```python
from build123d import *

# Parameters (mm, degrees)
F1_R      = 7.62
F2_DEPTH  = 8.9916
F3_R      = 3.175
F4_DEPTH  = 18.5
F7_DEPTH  = 21.5
F5_R      = 1.4351
F8_DEPTH  = 25.4
F11_DEPTH = 20
F12_R     = 2.54
F13_SIZE  = 2.54
F6_R      = 30.2514
F14_DEPTH = 2.032
F16_R     = 30.2514
F17_DEPTH = 2.032
F18_R     = 5.9079449729
F19_DEPTH = 3.81
F20_R     = 3.175
F20_R_2   = 1.016
F21_DEPTH = 20


# Not quite as in the source:
# - a feature of the source that left no trace in its solid (it failed there, or was rolled back) is left out
# - a feature names something its author has since deleted; it is built from what else it names


with BuildPart() as f2:
    # F1 (on Top) → F2 (new body)
    with BuildSketch(Plane.XY):
        with BuildLine():
            Line((14.3891, -27.8892), (14.3891, 5.7461149649))
            ThreePointArc((14.3891, 5.7461149649), (0, 15.494), (-14.3891, 5.7461149649))
            Line((-14.3891, 5.7461149649), (-14.3891, -27.8892))
            Line((-14.3891, -27.8892), (14.3891, -27.8892))
        make_face()
        Circle(F1_R, mode=Mode.SUBTRACT)
    extrude(amount=F2_DEPTH)


with BuildPart() as f4:
    # F3 (on Top) → F4 (new body)
    with BuildSketch(Plane.XY):
        Circle(F3_R)
    extrude(amount=F4_DEPTH)


with BuildPart() as f7:
    # F0 (on Top) → F7 (new body)
    with BuildSketch(Plane.XY):
        with BuildLine():
            Line((32.2834, -36.9807843447), (32.2834, 0))
            ThreePointArc((32.2834, 0), (0, 32.2834), (-32.2834, 0))
            Line((-32.2834, 0), (-32.2834, -36.9807843447))
            ThreePointArc((-32.2834, -36.9807843447), (-28.5636561211, -45.9610404657), (-19.5834, -49.6807843447))
            Line((-19.5834, -49.6807843447), (19.5834, -49.6807843447))
            ThreePointArc((19.5834, -49.6807843447), (28.5636561211, -45.9610404657), (32.2834, -36.9807843447))
        make_face()
    extrude(amount=F7_DEPTH)

    # F5 (on Top) → F8 (cut)
    with BuildSketch(Plane.XY):
        with Locations((-23.0124, 0)):
            Circle(F5_R)
        with Locations((23.0124, 0)):
            Circle(F5_R)
    extrude(amount=F8_DEPTH, mode=Mode.SUBTRACT)


with BuildPart() as f11_tool:
    # F10 (on Top) → F11 (new body)
    with BuildSketch(Plane.XY):
        with BuildLine():
            Line((-23.5020610966, -3.7882152164), (-27.6819982204, -3.7882152164))
            ThreePointArc((-27.6819982204, -3.7882152164), (-0.010778614, -27.9399979209), (27.6790671673, -3.8095722529))
            Line((27.6790671673, -3.8095722529), (23.0213215121, -3.8095722529))
            ThreePointArc((23.0213215121, -3.8095722529), (19.1556447136, -0.1037564295), (22.8138242261, 3.8070300236))
            ThreePointArc((22.8138242261, 3.8070300236), (22.9642316699, 3.81), (23.1146391137, 3.8070300236))
            Line((23.1146391137, 3.8070300236), (27.6794169447, 3.8070300236))
            ThreePointArc((27.6794169447, 3.8070300236), (-0.0092095477, 27.9399984822), (-27.6819206668, 3.7887818881))
            Line((-27.6819206668, 3.7887818881), (-23.4967496803, 3.7887818881))
            ThreePointArc((-23.4967496803, 3.7887818881), (-19.3067133937, 0.4041926109), (-22.688364657, -3.7882152164))
            ThreePointArc((-22.688364657, -3.7882152164), (-23.0952128768, -3.81), (-23.5020610966, -3.7882152164))
        make_face()
        with BuildLine():
            ThreePointArc((27.6790671673, -3.8095722529), (-0.010778614, -27.9399979209), (-27.6819982204, -3.7882152164))
            Line((-27.6819982204, -3.7882152164), (-27.6819982204, -34.7421456456))
            ThreePointArc((-27.6819982204, -34.7421456456), (-24.7062031172, -41.9263505425), (-17.5219982204, -44.9021456456))
            Line((-17.5219982204, -44.9021456456), (17.5190671673, -44.9021456456))
            ThreePointArc((17.5190671673, -44.9021456456), (24.7032720641, -41.9263505425), (27.6790671673, -34.7421456456))
            Line((27.6790671673, -34.7421456456), (27.6790671673, -3.8095722529))
        make_face()
        with BuildLine():
            Line((-22.688364657, -3.7882152164), (-23.5020610966, -3.7882152164))
            ThreePointArc((-23.5020610966, -3.7882152164), (-23.0952128768, -3.81), (-22.688364657, -3.7882152164))
        make_face()
        with BuildLine():
            ThreePointArc((23.1146391137, 3.8070300236), (22.9642316699, 3.81), (22.8138242261, 3.8070300236))
            Line((22.8138242261, 3.8070300236), (23.1146391137, 3.8070300236))
        make_face()
    extrude(amount=F11_DEPTH)


with BuildPart() as f2_1:
    add(f2.part)

    # F11: cut by f11_tool
    add(f11_tool.part, mode=Mode.SUBTRACT)


with BuildPart() as f4_1:
    add(f4.part)

    # F11: cut by f11_tool
    add(f11_tool.part, mode=Mode.SUBTRACT)


with BuildPart() as f7_1:
    add(f7.part)

    # F11: cut by f11_tool
    add(f11_tool.part, mode=Mode.SUBTRACT)

    # F12
    f12_edges = [f7_1.edges().sort_by_distance(p)[0] for p in [
        (0, 32.2834, 21.5),
        (32.2834, -18.490392, 21.5),
        (28.563656, -45.96104, 21.5),
        (0, -49.680784, 21.5),
        (-32.2834, -18.490392, 21.5),
        (-28.563656, -45.96104, 21.5),
    ]]
    fillet(f12_edges, radius=F12_R)

    # F13
    f13_edges = [f7_1.edges().sort_by_distance(p)[0] for p in [
        (-24.4475, 0, 21.5),
        (21.5773, 0, 21.5),
    ]]
    chamfer(f13_edges, length=F13_SIZE)

    # F6 (on Top) → F14 (cut)
    with BuildSketch(Plane.XY):
        Circle(F6_R)
    extrude(amount=F14_DEPTH, mode=Mode.SUBTRACT)

    # F16 (on Top) + F6 (on Top) → F17 (cut)
    with BuildSketch(Plane.XY):
        Circle(F16_R)
    with BuildSketch(Plane.XY):
        Circle(F6_R)
    extrude(amount=F17_DEPTH, mode=Mode.SUBTRACT)

    # F18 (on face) → F19 (cut)
    with BuildSketch(Plane.XZ.offset(49.6807843447)):
        with Locations((0, 9.48)):
            Circle(F18_R)
    extrude(amount=-F19_DEPTH, mode=Mode.SUBTRACT)

    # F20 (on face) → F21 (join, through all)
    with BuildSketch(Plane(origin=(0, 0, 20), x_dir=(1, 0, 0), z_dir=(0, 0, -1))):
        with Locations((17.5190671673, 34.7421456456)):
            Circle(F20_R)
        with Locations((17.5190671673, 34.7421456456)):
            Circle(F20_R_2, mode=Mode.SUBTRACT)
        with Locations((-17.5219982204, 34.7421456456)):
            Circle(F20_R)
        with Locations((-17.5219982204, 34.7421456456)):
            Circle(F20_R_2, mode=Mode.SUBTRACT)
    extrude(amount=F21_DEPTH)


solid = f7_1.part
```
Here's how the part is built. I have some questions about the finished solid (model axes, mm). A direction names the side the tool comes from. Give positions to 0.01 mm unless a question says otherwise; leave off trailing zeros. Order: outer loops, then holes, each group sorted by start corner. A loop starts at its lowest first (then second) coordinate and runs counter-clockwise, first axis right, second up. Notation, with made-up numbers: M 52,-33 L 64,-33 A32 cw 64,-6 Z; hole C -29.75,-18.75 d5. An arc over 180 degrees is marked long. Use a Markdown table: item, result. Add a question column.
1. I need wall thicknesses on probe 1 along X at (y, z) = (-9, 4.5); probe 2 along Y at (x, z) = (-1, 5.5); probe 3 along Y at (x, z) = (-19, 18.75). Which ranges of each line are inside material? Lowest first, please. Write a range as from..to.
2. Suppose I cut it at B-B (x = 0). List the corners of the cut face in (y, z) for me, and give its area (3 significant figures).
3. On a 3-axis mill with a long thin cutter (end or side, diameter ignored), from which of +Z, -Z, +X, -X, +Y, -Y can I reach the whole of each face in a straight line? I mean faces 5 (the flat face through (0, -8, 21.5)), 6 (the flat face through (0, -45.871, 10)), 7 (the cylindrical face through (-18.21, -31.643, 10.14)). Say none if no direction works.
4. If we mould it in two halves opening along X, with no side actions, what happens to faces 1 (the cylindrical face through (0.71, 32.276, 9.347)), 2 (the flat face through (17, -33, 0)), 3 (the flat face through (18, -35, 20)), 4 (the cylindrical face through (-31.559, -18.749, 20.736))? For each: +X half, -X half, draft (parallel to the pull), parting line (faces both ways), or undercut.
5. Suppose I cut it at A-A (z = 9.48). Give the number of separate pieces and of enclosed holes in the cut face, and give its area (3 significant figures).
6. For pin 1 Ø12.5 at (x, y) = (4.5, 14.5) entering from -Z; pin 2 Ø5.5 at (x, z) = (24.5, 9) entering from +Y; pin 3 Ø8 at (y, z) = (15.5, 18) entering from +X; pin 4 Ø2.5 at (x, y) = (23.01, 0) entering from -Z, each with a flat end and sliding along its axis, tell me the tip position at first contact or that it passes through.
Results list:
| question | item | result |
|---|---|---|
| 1 | probe 1 | x = -32.28..-27.68, 27.68..32.28 |
| 1 | probe 2 | y = -45.87..-44.9, 27.92..32.27 |
| 1 | probe 3 | y = -49.68..-44.79, -37.55..-31.93, 20.49..26.1 |
| 2 | outline | M -49.68,0 L -44.9,0 L -44.9,20 L 27.94,20 L 27.94,2.03 L 30.25,2.03 L 30.25,0 L 32.28,0 L 32.28,18.96 A2.54 ccw 29.74,21.5 L -47.14,21.5 A2.54 ccw -49.68,18.96 L -49.68,15.39 L -45.87,15.39 L -45.87,3.57 L -49.68,3.57 Z |
| 2 | area | 253 mm² |
| 3 | face 5 | +Z, +X, -X, +Y, -Y |
| 3 | face 6 | -Y |
| 3 | face 7 | -Z |
| 4 | face 1 | parting line |
| 4 | face 2 | draft |
| 4 | face 3 | undercut |
| 4 | face 4 | -X half |
| 5 | separate pieces | 3 |
| 5 | enclosed holes | 5 |
| 5 | area | 1,220 mm² |
| 6 | pin 1 | stops at z = 20 |
| 6 | pin 2 | stops at y = 23.86 |
| 6 | pin 3 | stops at x = 30.17 |
| 6 | pin 4 | passes through |
